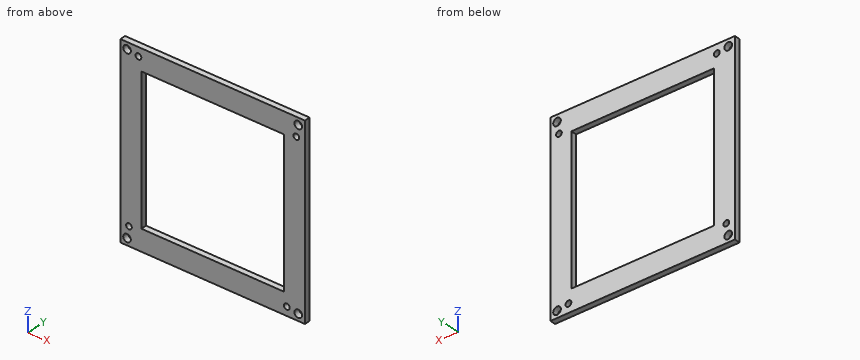
```python
from build123d import *

# Parameters (mm, degrees)
SKETCH1_W           = 97
SKETCH1_H           = 97
BOSS_EXTRUDE1_DEPTH = 3
SKETCH2_R           = 1.5
CUT_EXTRUDE4_DEPTH  = 138.211515552
SKETCH3_W           = 75
SKETCH3_H           = 75
CUT_EXTRUDE5_DEPTH  = 7
SKETCH4_R           = 2
CUT_EXTRUDE6_DEPTH  = 10


with BuildPart() as part:
    # Sketch1 → Boss-Extrude1 (new body)
    with BuildSketch(Plane(origin=(0, 0, 0), x_dir=(1, 0, 0), z_dir=(0, 1, 0))):
        with Locations((48.5, 48.5)):
            Rectangle(SKETCH1_W, SKETCH1_H)
    extrude(amount=BOSS_EXTRUDE1_DEPTH)

    # Sketch2 → Cut-Extrude4 (cut, through all)
    with BuildSketch(Plane(origin=(0, 3, 0), x_dir=(1, 0, 0), z_dir=(0, 1, 0))):
        with Locations(Location((4.5, 87.5, 0), (0, 0, 270))):
            Circle(SKETCH2_R)
        with Locations(Location((87.5, 92.5, 0), (0, 0, 270))):
            Circle(SKETCH2_R)
        with Locations(Location((92.5, 9.5, 0), (0, 0, 270))):
            Circle(SKETCH2_R)
        with Locations(Location((9.5, 4.5, 0), (0, 0, 270))):
            Circle(SKETCH2_R)
    extrude(amount=-CUT_EXTRUDE4_DEPTH, mode=Mode.SUBTRACT)

    # Sketch3 → Cut-Extrude5 (cut)
    with BuildSketch(Plane(origin=(0, 3, 0), x_dir=(1, 0, 0), z_dir=(0, 1, 0))):
        with Locations((48.5, 48.5)):
            Rectangle(SKETCH3_W, SKETCH3_H)
    extrude(amount=-CUT_EXTRUDE5_DEPTH, mode=Mode.SUBTRACT)

    # Sketch4 → Cut-Extrude6 (cut)
    with BuildSketch(Plane(origin=(0, 3, 0), x_dir=(1, 0, 0), z_dir=(0, 1, 0))):
        with Locations(Location((93.5, 3.5, 0), (0, 0, 270))):
            Circle(SKETCH4_R)
        with Locations(Location((3.5, 93.5, 0), (0, 0, 270))):
            Circle(SKETCH4_R)
        with Locations(Location((93.5, 93.5, 0), (0, 0, 270))):
            Circle(SKETCH4_R)
        with Locations(Location((3.5, 3.5, 0), (0, 0, 270))):
            Circle(SKETCH4_R)
    extrude(amount=-CUT_EXTRUDE6_DEPTH, mode=Mode.SUBTRACT)


solid = part.part
```
The model under review builds one solid part; all positions refer to its coordinate system, in mm. Round coordinates to 2 decimals unless told otherwise and drop trailing zeros. Write each loop counter-clockwise with the first axis right and the second up, starting at its lowest first coordinate (ties: lowest second). Pieces come first, ordered by that corner, then holes.
(1) Wall thickness on L1, parallel to Z at x = 65, y = 1.7; L2, parallel to X at y = 1.05, z = -13.5; L3, parallel to X at y = 1.45, z = -4.5: over which ranges is each line inside the solid? List them lowest first.
(2) We need section C-C on y = 2.35. Give the number of separate pieces and of enclosed holes in the cut face, and give its area (3 significant figures).
(3) Insertion check: pin 1 (3 mm diameter, centred on x = 3.5, z = -93.5, fed in from +Y). The pin has a flat end and moves straight along its axis. Give the tip position at first contact, or say it passes through.
(4) We need section A-A on x = 80.5. Give the boundary of the cut face in (y, z).
(5) We need section B-B on z = -69.5. Give the boundary of the cut face in (x, y), and give its area (3 significant figures).
Findings below:
1. L1: z = -97 to -86, -11 to 0
1. L2: x = 0 to 11, 86 to 97
1. L3: x = 0 to 1.77, 5.23 to 8, 11 to 91.77, 95.23 to 97
2. separate pieces: 1
2. enclosed holes: 9
2. area: 3,710 mm2
3. pin 1: passes through
4. outline: (0, -97) - (3, -97) - (3, -86) - (0, -86) - close; (0, -11) - (3, -11) - (3, 0) - (0, 0) - close
5. outline: (0, 0) - (11, 0) - (11, 3) - (0, 3) - close; (86, 0) - (97, 0) - (97, 3) - (86, 3) - close
5. area: 66.0 mm2
